Model file for the job. Use its own axes, mm. A direction names the side the tool comes from. Give positions to 0.01 mm unless a question says otherwise; leave off trailing zeros. Loops run counter-clockwise (first coordinate to the right, second up) from the corner with the lowest first, then second, coordinate; pieces in that order, holes last. Notation, with made-up numbers: M 86.5,2 L 136.5,2 A22 cw 136.5,33 Z; hole C 10,72.25 d4. An arc over 180 degrees is marked long. Answer in a Markdown table with one row per item.
Autodesk Inventor part; units mm, degrees
ref_plane "YZ Plane" through (0, 0, 0) normal (1, 0, 0) x (0, 1, 0)
ref_plane "XZ Plane" through (0, 0, 0) normal (0, 1, 0) x (-1, 0, 0)
ref_plane "XY Plane" through (0, 0, 0) normal (0, 0, 1) x (1, 0, 0)
sketch "Sketch1" plane through (0, 0, 0) normal (0, 1, 0) x (-1, 0, 0)
  line L0 (3.175, 0) -> (155.575, 0)
  line L1 (158.75, -3.175) -> (158.75, -161.925)
  line L2 (155.575, -165.1) -> (3.175, -165.1)
  line L3 (0, -161.925) -> (0, -3.175)
  arc A0 (158.75, -3.175) -> (155.575, 0) centre (155.575, -3.175) ccw
  arc A1 (155.575, -165.1) -> (158.75, -161.925) centre (155.575, -161.925) ccw
  arc A2 (0, -161.925) -> (3.175, -165.1) centre (3.175, -161.925) ccw
  arc A3 (3.175, 0) -> (0, -3.175) centre (3.175, -3.175) ccw
  point P0 (0, 0)
  point P1 (158.75, -165.1)
  point P2 (158.75, 0)
  point P3 (0, -165.1)
  dimension "d0" = 158.75
  dimension "d1" = 165.1
  dimension "d2" = 3.175
  dimension "d3" = 3.175
  dimension "d4" = 3.175
  dimension "d5" = 3.175
extrude "Extrusion1" add sketch "Sketch1" along normal blind 82.55
sketch "Sketch2" plane through (0, 0, 0) normal (0, -1, 0) x (1, 0, 0)
  line L0 (-3.175, -165.1) -> (-155.575, -165.1)
  line L1 (-6.5142, -165.1) -> (0, -165.1)
  line L2 (0, -158.9917) -> (0, -165.1)
  line L3 (0, -165.1) -> (-7.9375, -165.1)
  line L4 (-7.9375, -165.1) -> (-7.9375, -157.1625)
  line L5 (-7.9375, -157.1625) -> (0, -157.1625)
  line L6 (0, -157.1625) -> (0, -165.1)
  line L7 (-7.9375, -157.1625) -> (-149.225, -157.1625)
  line L8 (-7.9375, -157.1625) -> (-7.9375, -41.275)
  line L9 (-7.9375, -41.275) -> (-42.5857, -6.6268)
  line L10 (-7.9375, -41.275) -> (41.0625, -41.275) construction
  point P0 (0, 0)
  dimension "d8" = 7.9375
  dimension "d9" = 7.9375
  dimension "d10" = 141.2875
  dimension "d11" = 115.8875
  dimension "d12" = 49
  dimension "d13" = 135
hole "Hole1" at (-42.5857, 0, -6.6268) at (-7.9375, 0, -41.275) at (-7.9375, 0, -157.1625) at (-149.225, 0, -157.1625) direction (0, 1, 0) diameter 4.7625 end through all
sketch "Sketch7" plane through (-3.175, 0, -165.1) normal (0, 0, -1) x (-1, 0, 0)
  line L0 (0, 0) -> (0, 82.55)
  line L1 (0, 82.55) -> (44.45, 82.55)
  line L2 (152.4, 82.55) -> (0, 82.55)
  line L3 (0, 82.55) -> (44.45, 82.55) construction
  line L4 (44.45, 82.55) -> (107.95, 82.55)
  line L5 (107.95, 82.55) -> (107.95, 6.35)
  line L6 (107.95, 6.35) -> (44.45, 6.35)
  line L7 (44.45, 6.35) -> (44.45, 82.55)
  line L8 (44.45, 6.35) -> (0, 82.55)
  line L9 (107.95, 6.35) -> (152.4, 82.55)
  line L10 (107.95, 82.55) -> (152.4, 82.55)
  point P0 (-3.175, 0)
  dimension "d22" = 44.45
  dimension "d23" = 0
  dimension "d24" = 63.5
  dimension "d25" = 76.2
sketch "Sketch8" plane through (0, 0, -3.175) normal (1, 0, 0) x (0, 0, -1)
  line L0 (0, 82.55) -> (-3.175, 82.55)
  line L1 (0, 82.55) -> (158.75, 82.55)
  line L2 (23.1966, 82.55) -> (161.925, 6.35)
  line L3 (161.925, 0) -> (161.925, 82.55)
  point P0 (-3.175, 0)
sweep "Sweep1" cut profiles "Sketch7" path "Sketch8" path curves L2
sketch "Sketch9" plane through (0, 82.55, 0) normal (0, 1, 0) x (1, 0, 0)
  line L0 (-3.175, 165.1) -> (-155.575, 165.1)
  line L1 (0, 3.175) -> (0, 161.925)
  line L2 (-13.8845, 165.1) -> (0, 165.1)
  line L3 (0, 165.1) -> (0, 151.6388)
  line L4 (0, 151.6388) -> (-13.8845, 151.6388)
  line L5 (-13.8845, 151.6388) -> (-13.8845, 165.1)
  line L6 (-143.876, 151.6388) -> (-158.75, 151.6388)
  line L7 (-158.75, 151.6388) -> (-158.75, 165.1)
  line L8 (-158.75, 165.1) -> (-143.876, 165.1)
  line L9 (-143.876, 165.1) -> (-143.876, 151.6388)
  line L10 (0, 3.175) -> (0, 161.925)
  line L11 (-15.8979, 48.8027) -> (0, 48.8027)
  line L12 (0, 48.8027) -> (0, 34.9422)
  line L13 (0, 34.9422) -> (-15.8979, 34.9422)
  line L14 (-15.8979, 34.9422) -> (-15.8979, 48.8027)
  line L15 (-47.625, 0) -> (-47.625, 165.1)
  line L16 (-35.1821, 14.6536) -> (-47.625, 14.6536)
  line L17 (-47.625, 14.6536) -> (-47.625, 0)
  line L18 (-47.625, 0) -> (-35.1821, 0)
  line L19 (-35.1821, 0) -> (-35.1821, 14.6536)
  point P0 (0, 0)
  point P1 (0, 48.8027)
extrude "Extrusion2" cut sketch "Sketch9" against normal blind 16.51 contours L2 L3 L1 L4 L5 L0 | L1 L13 L14 L11 | L16 L19 L18 L15
extrude "Extrusion3" cut sketch "Sketch9" against normal blind 80.01 contours L9 L6 L7 L8 L0
sketch "Sketch11" plane through (-3.175, 0, -165.1) normal (0, 0, -1) x (-1, 0, 0)
  line L0 (44.45, 82.55) -> (44.45, 6.35)
  line L1 (107.95, 6.35) -> (44.45, 6.35)
  line L2 (44.45, 6.35) -> (107.95, 6.35)
  line L3 (107.95, 6.35) -> (107.95, 3.175)
  line L4 (107.95, 3.175) -> (44.45, 3.175)
  line L5 (44.45, 3.175) -> (44.45, 6.35)
  line L6 (44.45, 6.35) -> (9.6308, 66.04)
  line L7 (21.1649, 46.2673) -> (46.3021, 3.175)
  line L8 (46.3021, 3.175) -> (43.5596, 1.5752)
  line L9 (43.5596, 1.5752) -> (18.4224, 44.6675)
  line L10 (18.4224, 44.6675) -> (21.1649, 46.2673)
  line L11 (140.701, 62.4945) -> (107.95, 6.35)
  line L12 (131.2351, 46.2673) -> (106.0979, 3.175)
  line L13 (106.0979, 3.175) -> (108.8404, 1.5752)
  line L14 (108.8404, 1.5752) -> (133.9776, 44.6675)
  line L15 (133.9776, 44.6675) -> (131.2351, 46.2673)
  point P0 (-3.175, 0)
  dimension "d40" = 3.175
  dimension "d41" = 3.175
  dimension "d42" = 3.175
extrude "Extrusion5" add sketch "Sketch11" along normal blind 25.4
properties part number "pipet tip trough"
Q1. 3-axis set-ups, long thin cutter, end or side, ignore diameter. For faces 1 (the face through (-124.41, 22.82, -177.62)), 2 (the face through (-36.145, 26.029, -177.622)), 3 (the face through (-34.34, 22.82, -177.62)), 4 (the face through (-15.898, 74, -42)): which of +Z, -Z, +X, -X, +Y, -Y reach the whole face in a straight line?
Reported:
| item | result |
|---|---|
| face 1 | -Z, -X, -Y |
| face 2 | -Z, +Y |
| face 3 | -Z, +X, -Y |
| face 4 | +X, +Y |
Q2. Drop flat-ended pins along their axis: pin 1 (6.5 mm diameter, centred on x = -4.5, z = -158.5, fed in from +Y); pin 2 (6.5 mm diameter, centred on x = -151.5, z = -156.5, fed in from +Y); pin 3 (17.5 mm diameter, centred on x = -8.5, y = 74, fed in from -Z); pin 4 (3 mm diameter, centred on x = -42.59, z = -6.63, fed in from -Y) (3 decimals). Give the stop position or say it passes through.
Reported:
| item | result |
|---|---|
| pin 1 | y = 66.04 |
| pin 2 | y = 2.54 |
| pin 3 | z = -165.1 |
| pin 4 | through |
Q3. Probe probe 1 along Z at (x, y) = (-140.5, 45); probe 2 along X at (y, z) = (12.5, -161); probe 3 along Y at (x, z) = (-58, -172) (3 decimals). List the from-to ranges inside material, lowest first.
Reported:
| item | result |
|---|---|
| probe 1 | -165.1 to 0 |
| probe 2 | -143.88 to -113.4, -45.35 to 0 |
| probe 3 | 3.175 to 6.35 |
Q4. Mould opens along X. For faces 5 (the face through (-13.884, 68, -154)), 6 (the face through (-5.613, 33.482, -156.646)), 7 (the face through (-35.182, 74, -7)), 8 (the face through (-79, 6, -190.5)) say: released by +X, released by -X, zero draft, split by the parting line, or undercut.
Reported:
| item | result |
|---|---|
| face 5 | released by +X |
| face 6 | undercut |
| face 7 | undercut |
| face 8 | zero draft |
Q5. Saw through at C-C (x = -140.5). Give the cut face in (y, z).
Reported:
| item | result |
|---|---|
| outline | M 0,-165.1 L 56.71,-165.1 L 82.55,-118.05 L 82.55,0 L 0,0 Z |
Q6. Saw through at B-B (y = 54). Give the number of separate pieces and of enclosed holes in the cut face, and give its area (3 significant figures).
Reported:
| item | result |
|---|---|
| separate pieces | 1 |
| enclosed holes | 3 |
| area | 18,000 mm² |
